Check sheet for the modelled part. Datum: model origin and axes. Units: mm. Give positions to 0.01 mm unless a question says otherwise; leave off trailing zeros. Write each loop counter-clockwise with the first axis right and the second up, starting at its lowest first coordinate (ties: lowest second). Pieces come first, ordered by that corner, then holes. Notation, with made-up numbers: (40.25, 6) -> (95.25, 6) arc R26 cw to (95.25, 35) -> close; hole circle Ø6 at (32.5, -25.75). An arc over 180 degrees is marked (long way). Use a Markdown table: item, result. Add a question column.
1. Gauge pin test, flat ends, axial feed: P1, Ø5, axis at x = 1, z = 45, coming from the -Y side; P2, Ø6.5, axis at y = 0, z = 26, coming from the -X side; P3, Ø3, axis at x = -2, z = 103, coming from the +Y side; P4, Ø6.5, axis at x = 2, z = 112, coming from the -Y side. Record the tip position at first contact, or that the pin passes through.
2. Scan lines: probe 1 along Y at (x, z) = (-1.5, 108); probe 2 along Y at (x, z) = (5, 73); probe 3 along Y at (x, z) = (2.25, 32). Record each from-to range of solid material in increasing order. Write a range as [from, to].
3. Cross-section at A-A (y = 0). Enter the section's corners in (x, z), then the cut area to 3 significant figures.
4. Cross-section at B-B (z = 56.4). Count the separate pieces of the cut face and the enclosed holes in it, then the cut area to 3 significant figures.
from build123d import *

# Parameters (mm, degrees)
EXTRUDE_1_DEPTH           = 160
HOLE_WIZARD_8_0_8_1_D     = 8
HOLE_WIZARD_8_0_8_2_D     = 8
HOLE_WIZARD_8_0_8_2_DEPTH = 8
HOLE_WIZARD_8_0_8_2_TIP   = 2.403442476
HOLE_WIZARD_12_0_12_2_D   = 12
HOLE_WIZARD_5_5_5_5_1_D   = 5.5
HOLE_WIZARD_5_5_5_5_2_D   = 5.5
HOLE_WIZARD_5_5_5_5_3_D   = 5.5
HOLE_WIZARD_5_5_5_5_4_D   = 5.5
HOLE_WIZARD_M5_1_D        = 4.2
HOLE_WIZARD_M5_2_D        = 4.2


with BuildPart() as part:
    # Sketch1 → 凸台-拉伸1 (new body)
    with BuildSketch(Plane.XY):
        with BuildLine():
            Line((-9, 40), (-4.15, 40))
            Line((-4.15, 40), (-4.15, 37))
            Line((-4.15, 37), (-7.05, 37))
            Line((-7.05, 37), (-7.05, 30))
            Line((-7.05, 30), (7.05, 30))
            Line((7.05, 30), (7.05, 37))
            Line((7.05, 37), (4.15, 37))
            Line((4.15, 37), (4.15, 40))
            Line((4.15, 40), (9, 40))
            ThreePointArc((9, 40), (9.707106781, 39.707106781), (10, 39))
            Line((10, 39), (10, 24.15))
            Line((10, 24.15), (6, 24.15))
            Line((6, 24.15), (6, 27.05))
            Line((6, 27.05), (0, 27.05))
            Line((0, 27.05), (0, 24.15))
            Line((0, 24.15), (-4, 24.15))
            Line((-4, 24.15), (-4, 15.85))
            Line((-4, 15.85), (0, 15.85))
            Line((0, 15.85), (0, 12.95))
            Line((0, 12.95), (6, 12.95))
            Line((6, 12.95), (6, 15.85))
            Line((6, 15.85), (10, 15.85))
            Line((10, 15.85), (10, -15.85))
            Line((10, -15.85), (6, -15.85))
            Line((6, -15.85), (6, -12.95))
            Line((6, -12.95), (0, -12.95))
            Line((0, -12.95), (0, -15.85))
            Line((0, -15.85), (-4, -15.85))
            Line((-4, -15.85), (-4, -24.15))
            Line((-4, -24.15), (0, -24.15))
            Line((0, -24.15), (0, -27.05))
            Line((0, -27.05), (6, -27.05))
            Line((6, -27.05), (6, -24.15))
            Line((6, -24.15), (10, -24.15))
            Line((10, -24.15), (10, -39))
            ThreePointArc((10, -39), (9.707106781, -39.707106781), (9, -40))
            Line((9, -40), (4.15, -40))
            Line((4.15, -40), (4.15, -37))
            Line((4.15, -37), (7.05, -37))
            Line((7.05, -37), (7.05, -30))
            Line((7.05, -30), (-7.05, -30))
            Line((-7.05, -30), (-7.05, -37))
            Line((-7.05, -37), (-4.15, -37))
            Line((-4.15, -37), (-4.15, -40))
            Line((-4.15, -40), (-9, -40))
            ThreePointArc((-9, -40), (-9.707106781, -39.707106781), (-10, -39))
            Line((-10, -39), (-10, -4.15))
            Line((-10, -4.15), (-6, -4.15))
            Line((-6, -4.15), (-6, -7.05))
            Line((-6, -7.05), (0, -7.05))
            Line((0, -7.05), (0, -4.15))
            Line((0, -4.15), (4, -4.15))
            Line((4, -4.15), (4, 4.15))
            Line((4, 4.15), (0, 4.15))
            Line((0, 4.15), (0, 7.05))
            Line((0, 7.05), (-6, 7.05))
            Line((-6, 7.05), (-6, 4.15))
            Line((-6, 4.15), (-10, 4.15))
            Line((-10, 4.15), (-10, 39))
            ThreePointArc((-10, 39), (-9.707106781, 39.707106781), (-9, 40))
        make_face()
    extrude(amount=EXTRUDE_1_DEPTH)

    # Ø8.0 (8) 直径孔1 (through all)
    with Locations(Plane(origin=(10, 0, 0), x_dir=(0, 0, -1), z_dir=(1, 0, 0))):
        with Locations((-134, 0)):
            Hole(HOLE_WIZARD_8_0_8_1_D / 2)

    # Ø8.0 (8) 直径孔2
    with Locations(Plane(origin=(10, 0, 0), x_dir=(0, 0, -1), z_dir=(1, 0, 0))):
        with Locations((-26, 0)):
            Hole(HOLE_WIZARD_8_0_8_2_D / 2, depth=HOLE_WIZARD_8_0_8_2_DEPTH)
            with Locations((0, 0, -(HOLE_WIZARD_8_0_8_2_DEPTH + HOLE_WIZARD_8_0_8_2_TIP / 2))):  # 118° drill point
                Cone(0, HOLE_WIZARD_8_0_8_2_D / 2, HOLE_WIZARD_8_0_8_2_TIP, mode=Mode.SUBTRACT)

    # Ø12.0 (12) 直径孔2 (through all)
    with Locations(Plane(origin=(10, 0, 0), x_dir=(0, 0, -1), z_dir=(1, 0, 0))):
        with Locations((-80, 0)):
            Hole(HOLE_WIZARD_12_0_12_2_D / 2)

    # Ø5.5 (5.5) 直径孔1 (through all)
    with Locations(Plane.ZY.offset(10)):
        with Locations((103.6, -20)):
            Hole(HOLE_WIZARD_5_5_5_5_1_D / 2)

    # Ø5.5 (5.5) 直径孔2 (through all)
    with Locations(Plane.ZY.offset(10)):
        with Locations((56.4, -20)):
            Hole(HOLE_WIZARD_5_5_5_5_2_D / 2)

    # Ø5.5 (5.5) 直径孔3 (through all)
    with Locations(Plane.ZY.offset(10)):
        with Locations((103.6, 20)):
            Hole(HOLE_WIZARD_5_5_5_5_3_D / 2)

    # Ø5.5 (5.5) 直径孔4 (through all)
    with Locations(Plane.ZY.offset(10)):
        with Locations((56.4, 20)):
            Hole(HOLE_WIZARD_5_5_5_5_4_D / 2)

    # M5 螺纹孔1 (through all)
    with Locations(Plane.ZY.offset(10)):
        with Locations((80, -18.25)):
            Hole(HOLE_WIZARD_M5_1_D / 2)

    # M5 螺纹孔2 (through all)
    with Locations(Plane.ZY.offset(10)):
        with Locations((80, 18.25)):
            Hole(HOLE_WIZARD_M5_2_D / 2)


solid = part.part
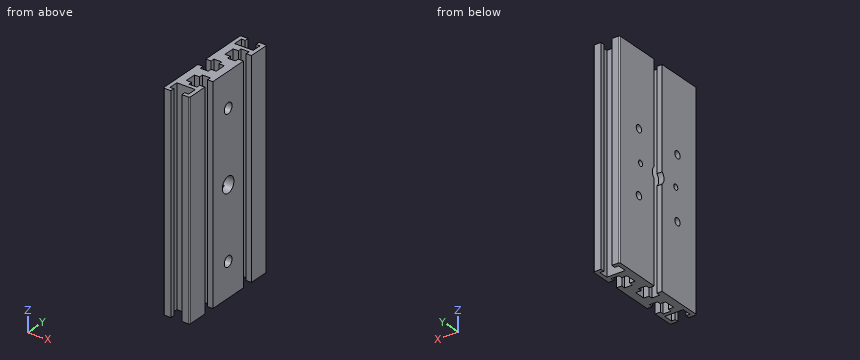
Worked answers:
| question | item | result |
|---|---|---|
| 1 | P1 | stops at y = -30 |
| 1 | P2 | passes through |
| 1 | P3 | stops at y = 30 |
| 1 | P4 | stops at y = -40 |
| 2 | probe 1 | y = [-30, -24.15], [-15.85, -7.05], [7.05, 15.85], [24.15, 30] |
| 2 | probe 2 | y = [-40, -37], [-30, -27.05], [-12.95, 12.95], [27.05, 30], [37, 40] |
| 2 | probe 3 | y = [-30, -27.05], [-12.95, -4.15], [4.15, 12.95], [27.05, 30] |
| 3 | outline | (4, 0) -> (10, 0) -> (10, 22) -> (4, 22) -> close; (4, 30) -> (10, 30) -> (10, 74) -> (4, 74) -> close; (4, 86) -> (10, 86) -> (10, 130) -> (4, 130) -> close; (4, 138) -> (10, 138) -> (10, 160) -> (4, 160) -> close |
| 3 | area | 792 mm² |
| 4 | separate pieces | 3 |
| 4 | enclosed holes | 0 |
| 4 | area | 833 mm² |
